Geometry check sheet. Reference: the model listing, model coordinates, mm. Round coordinates to 2 decimals unless told otherwise and drop trailing zeros. Order: outer loops, then holes, each group sorted by start corner. A loop starts at its lowest first (then second) coordinate and runs counter-clockwise, first axis right, second up.
(1) Go/stop test with flat-tipped pins: pin 1 (3.5 mm diameter, centred on x = -39.56, y = 97.17, fed in from -Z); pin 2 (5 mm diameter, centred on x = -39.56, y = -80.63, fed in from -Z). Record where each tip stops, or that it passes through.
(2) Sectioned sample at A-A (z = 1.25). Record the boundary of the cut face in (x, y), plus the area to 3 significant figures.
(3) Material ranges on line 1 along Y through (x, z) = (-42, 0.55); line 2 along X through (y, z) = (-34, 1.05); line 3 along Y through (x, z) = (-2, 1.15), recorded low to high.
(4) Sectioned sample at C-C (y = 53). Record the boundary of the cut face in (x, z).
(5) Sectioned sample at B-B (x = 2.5). Record the boundary of the cut face in (y, z), plus the area to 3 significant figures.
Autodesk Inventor part; units mm, degrees
ref_plane "YZ Plane" through (0, 0, 0) normal (1, 0, 0) x (0, 1, 0)
ref_plane "XZ Plane" through (0, 0, 0) normal (0, 1, 0) x (-1, 0, 0)
ref_plane "XY Plane" through (0, 0, 0) normal (0, 0, 1) x (1, 0, 0)
sketch "Sketch1" plane through (0, 0, 0) normal (0, 0, 1) x (1, 0, 0)
  circle A0 centre (-39.5621, -80.6318) radius 2.1844
  circle A1 centre (-14.1621, -80.6318) radius 2.1844
  circle A2 centre (-14.1621, 97.1682) radius 2.1844
  circle A3 centre (-39.5621, 97.1682) radius 2.1844
  arc A4 (19.2671, -81.2453) -> (23.3688, -75.2127) centre (18.394, -76.2409) ccw
  line L0 (19.2671, -81.2453) -> (-13.0707, -86.8873)
  arc A5 (14.8318, 8.2682) -> (23.3688, -75.2127) centre (427.2689, 8.2682) ccw
  arc A6 (23.3688, 91.749) -> (14.8318, 8.2682) centre (427.2689, 8.2682) ccw
  arc A7 (23.3688, 91.749) -> (19.2671, 97.7816) centre (18.394, 92.7772) ccw
  line L1 (19.2671, 97.7816) -> (-13.0707, 103.4237)
  line L2 (-39.5621, -86.9818) -> (-14.1621, -86.9818)
  line L3 (-14.1621, 103.5182) -> (-39.5621, 103.5182)
  line L4 (-45.9121, -80.6318) -> (-45.9121, 97.1682)
  arc A8 (-45.9121, -80.6318) -> (-39.5621, -86.9818) centre (-39.5621, -80.6318) ccw
  arc A9 (-14.1621, -86.9818) -> (-13.0707, -86.8873) centre (-14.1621, -80.6318) ccw
  arc A10 (-13.0707, 103.4237) -> (-14.1621, 103.5182) centre (-14.1621, 97.1682) ccw
  arc A11 (-39.5621, 103.5182) -> (-45.9121, 97.1682) centre (-39.5621, 97.1682) ccw
  point P0 (0, 0)
  dimension "d0" = 5.08
extrude "Extrusion1" add sketch "Sketch1" along normal blind 1.5875
properties part number "wedge"
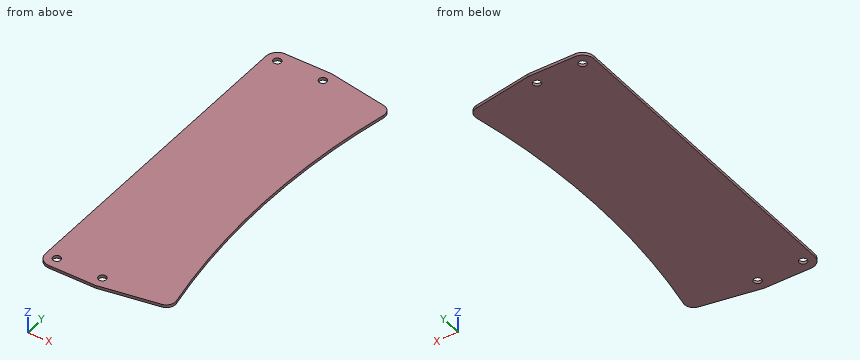
Answer below:
1. pin 1: passes through
1. pin 2: stops at z = 0
2. outline: (-45.91, -80.63) arc R6.35 ccw to (-39.56, -86.98) - (-14.16, -86.98) arc R6.35 ccw to (-13.07, -86.89) - (19.27, -81.25) arc R5.08 ccw to (23.37, -75.21) arc R412.44 cw to (14.83, 8.27) arc R412.44 cw to (23.37, 91.75) arc R5.08 ccw to (19.27, 97.78) - (-13.07, 103.42) arc R6.35 ccw to (-14.16, 103.52) - (-39.56, 103.52) arc R6.35 ccw to (-45.91, 97.17) - close; hole circle Ø4.37 at (-39.56, -80.63); hole circle Ø4.37 at (-39.56, 97.17); hole circle Ø4.37 at (-14.16, -80.63); hole circle Ø4.37 at (-14.16, 97.17)
2. area: 11,900 mm2
3. line 1: y = -86.5 to 103.03
3. line 2: x = -45.91 to 17
3. line 3: y = -84.96 to 101.49
4. outline: (-45.91, 0) - (17.26, 0) - (17.26, 1.59) - (-45.91, 1.59) - close
5. outline: (-84.17, 0) - (100.71, 0) - (100.71, 1.59) - (-84.17, 1.59) - close
5. area: 293 mm2
